The listing builds one solid part. Answer for the finished solid, in the listing's coordinates (mm). Face numbers are marked on the shaded views. A direction names the side the tool comes from. Round coordinates to 2 decimals unless told otherwise and drop trailing zeros. Write each loop counter-clockwise with the first axis right and the second up, starting at its lowest first coordinate (ties: lowest second). Pieces come first, ordered by that corner, then holes. Notation, with made-up numbers: M -34,36 L -25,36 A20 ccw -25,67 Z; hole C 9.25,46.5 d9. An arc over 180 degrees is marked long. One line per item, written item: value. Start each with the question number.
(1) For a pull along Z with two mould halves and no side action, classify the marked faces 4, 5, 6 and 7 as released by +Z, released by -Z, zero draft, split by the parting line, or undercut.
(2) Section D-D (y = -11.25) is taken. Determine the outline of the cut face in (x, z), plus the area to 3 significant figures.
(3) Given P1, Ø1.1, axis at x = -8.5, y = -10.5, coming from the -Z side; P2, Ø3, axis at x = 0, y = -7.5, coming from the -Z side, each flat-ended and moving along its own axis, determine where each tip first touches the part or whether it passes through.
(4) For the marked faces 1, 2 and 3, determine the directions among +Z, -Z, +X, -X, +Y, -Y from which every point of the face is accessible in a straight line to the end or side of a thin tool.
(5) Section A-A (x = 0) is taken. Determine the outline of the cut face in (y, z).
(6) Consider probe 1 along X at (y, z) = (-9.5, 7.5); probe 2 along Y at (x, z) = (0, 1.55); probe 3 along Z at (x, y) = (-0.75, -11.5). Determine where each line is inside the solid, lowest interval first.
(7) Section B-B (y = -7.5) is taken. Determine the outline of the cut face in (x, z).
(8) Section C-C (z = 7.25) is taken. Determine the outline of the cut face in (x, y), plus the area to 3 significant figures.
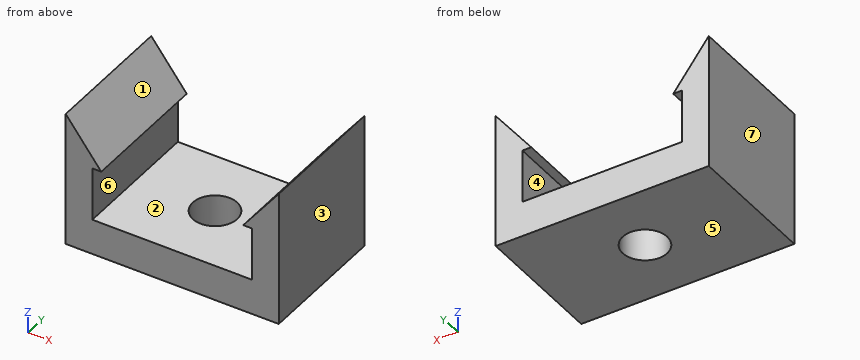
```python
from build123d import *

# Parameters (mm, degrees)
F1_DEPTH = 15
F4_D     = 5


with BuildPart() as f1:
    # F0 (on Front) → F1 (new body)
    with BuildSketch(Plane.XZ):
        Polygon((0, 0), (12, 0), (12, 15.199336), (8, 10), (9, 10), (9, 4), (0, 4), align=None)
    extrude(amount=F1_DEPTH)

    # F2: F1 across face


with BuildPart() as f1_1:
    add(f1.part)
    add(f1.part.mirror(Plane(origin=(0, -7.5, 2), x_dir=(0, -1, 0), z_dir=(-1, 0, 0))))

    # F4 (through all)
    with Locations(Plane.XY.offset(4)):
        with Locations((0, -7.5)):
            Hole(F4_D / 2)


solid = f1_1.part
```
Recorded:
1. face 4: undercut
1. face 5: released by -Z
1. face 6: undercut
1. face 7: zero draft
2. outline: M -12,0 L 12,0 L 12,15.2 L 8,10 L 9,10 L 9,4 L -9,4 L -9,10 L -8,10 L -12,15.2 Z
2. area: 153 mm2
3. P1: stops at z = 0
3. P2: passes through
4. face 1: +Z, +Y, -Y
4. face 2: +Y, -Y
4. face 3: +Z, -Z, +X, +Y, -Y
5. outline: M -15,0 L -10,0 L -10,4 L -15,4 Z; M -5,0 L 0,0 L 0,4 L -5,4 Z
6. probe 1: x = -12 to -9, 9 to 12
6. probe 2: y = -15 to -10, -5 to 0
6. probe 3: z = 0 to 4
7. outline: M -12,0 L -2.5,0 L -2.5,4 L -9,4 L -9,10 L -8,10 L -12,15.2 Z; M 2.5,0 L 12,0 L 12,15.2 L 8,10 L 9,10 L 9,4 L 2.5,4 Z
8. outline: M -12,-15 L -9,-15 L -9,0 L -12,0 Z; M 9,-15 L 12,-15 L 12,0 L 9,0 Z
8. area: 90.0 mm2
